```python
from build123d import *

# Parameters (mm, degrees)
SKETCH1_W           = 50.8
SKETCH1_H           = 50.8
BOSS_EXTRUDE1_DEPTH = 201.72011345
SHELL1_T            = -3.175
SKETCH2_R           = 2.4892
CUT_EXTRUDE3_DEPTH  = 215.13146469
SKETCH3_R           = 2.4892
CUT_EXTRUDE2_DEPTH  = 215.13146469
LPATTERN1_COUNT     = 8
LPATTERN1_PITCH     = 25.4


with BuildPart() as part:
    # Sketch1 → Boss-Extrude1 (new body)
    with BuildSketch(Plane(origin=(0, 0, 0), x_dir=(0, 0, -1), z_dir=(1, 0, 0))):
        with Locations((25.4, 25.4)):
            Rectangle(SKETCH1_W, SKETCH1_H)
    extrude(amount=BOSS_EXTRUDE1_DEPTH)

    # Shell1
    shell1_openings = [part.faces().sort_by_distance(p)[0] for p in [
        (201.72011345, 25.4, -25.4),
        (0, 25.4, -25.4),
    ]]
    offset(amount=SHELL1_T, openings=shell1_openings, kind=Kind.INTERSECTION)

    # Sketch2 → Cut-Extrude3 (cut, through all)
    with BuildSketch(Plane(origin=(0, 0, -50.8), x_dir=(-1, 0, 0), z_dir=(0, 0, -1))):
        with Locations((-195.262511684, 38.1)):
            Circle(SKETCH2_R)
        with Locations((-195.262511684, 12.7)):
            Circle(SKETCH2_R)
    cut_extrude3 = extrude(amount=-CUT_EXTRUDE3_DEPTH, mode=Mode.SUBTRACT)

    # Sketch3 → Cut-Extrude2 (cut, through all)
    with BuildSketch(Plane.XZ):
        with Locations(Location((195.262511684, -12.7, 0), (0, 0, 270))):
            Circle(SKETCH3_R)
        with Locations(Location((195.262511684, -38.1, 0), (0, 0, 270))):
            Circle(SKETCH3_R)
    cut_extrude2 = extrude(amount=-CUT_EXTRUDE2_DEPTH, mode=Mode.SUBTRACT)

    # LPattern1: Cut-Extrude3, Cut-Extrude2 ×8
    with Locations(*[(-i * LPATTERN1_PITCH, 0, 0) for i in range(1, LPATTERN1_COUNT)]):
        add(cut_extrude3, mode=Mode.SUBTRACT)
        add(cut_extrude2, mode=Mode.SUBTRACT)


solid = part.part
```
Geometry check sheet. Reference: the model listing, model coordinates, mm. Round coordinates to 2 decimals unless told otherwise and drop trailing zeros. Order: outer loops, then holes, each group sorted by start corner. A loop starts at its lowest first (then second) coordinate and runs counter-clockwise, first axis right, second up. Notation, with made-up numbers: (35.5, 7) - (56.5, 7) arc R10 cw to (56.5, 13) - close; hole circle Ø6 at (67, -5). An arc over 180 degrees is marked (long way). Use a Markdown table: item, result. Add a question column.
(1) Material ranges on line 1 along Z through (x, y) = (170.5, 5.5) (3 decimals); line 2 along Y through (x, z) = (178, -34.5) (3 decimals), recorded low to high. Write a range as [from, to].
(2) Sectioned sample at A-A, the plane z = -44. Enter the section's corners in (x, y) (3 decimals).
(3) Depth check by flat-ended pin: pin 1 (8 mm diameter, centred on x = 149, y = 33.5, fed in from +Z). Enter the tip coordinate at first touch or a pass-through.
(4) Sectioned sample at B-B, the plane y = 17.5. Enter the section's corners in (x, z) (3 decimals), and give its area (3 significant figures).
(5) Release check for a two-part mould opening along Y. For faces 1 (the cylindrical face through (197.73, 49.19, -12.38)), 2 (the flat face through (99, 47.625, -25)), 3 (the cylindrical face through (192.89, 13.45, -1.61)) record: pulls with the +Y half, pulls with the -Y half, needs draft (parallel to the pull), parting line crosses it, or undercut.
(6) Sectioned sample at C-C, the plane x = 34.5. Enter the section's corners in (y, z) (3 decimals).
Answers below:
| question | item | result |
|---|---|---|
| 1 | line 1 | [-50.8, -47.625], [-3.175, 0] |
| 1 | line 2 | [0, 3.175], [47.625, 50.8] |
| 2 | outline | (0, 0) - (201.72, 0) - (201.72, 3.175) - (0, 3.175) - close; (0, 47.625) - (201.72, 47.625) - (201.72, 50.8) - (0, 50.8) - close |
| 3 | pin 1 | z = 0 |
| 4 | outline | (0, -50.8) - (201.72, -50.8) - (201.72, -47.625) - (0, -47.625) - close; (0, -3.175) - (201.72, -3.175) - (201.72, 0) - (0, 0) - close |
| 4 | area | 1,280 mm² |
| 5 | face 1 | needs draft |
| 5 | face 2 | undercut |
| 5 | face 3 | undercut |
| 6 | outline | (0, -50.8) - (50.8, -50.8) - (50.8, 0) - (0, 0) - close; hole (3.175, -47.625) - (47.625, -47.625) - (47.625, -3.175) - (3.175, -3.175) - close |
